from build123d import *

# Parameters (mm, degrees)
EXTRUDE_1_DEPTH          = 2.5
EXTRUDE_1_DEPTH_BACK     = 2.5
SKETCH_1_W               = 10
SKETCH_1_H               = 5
EXTRUDE_3_DEPTH          = 1
EXTRUDE_3_DEPTH_BACK     = 1
SKETCH_2_6_R             = 0.5
CUT_EXTRUDE_1_DEPTH      = 0.5
CUT_EXTRUDE_1_DEPTH_BACK = 0.5
SKETCH_2_R               = 0.5


with BuildPart() as part:
    # Sketch 1 → Extrude 1 (new, two sides: drawn at the far end of the back side and taken through both)
    with BuildSketch(Plane.XY.offset(-EXTRUDE_1_DEPTH_BACK)):
        with Locations((5, 2.5)):
            Rectangle(SKETCH_1_W, SKETCH_1_H)
    extrude(amount=EXTRUDE_1_DEPTH + EXTRUDE_1_DEPTH_BACK)

    # Sketch 2_6 → Extrude 3 (add, two sides: drawn at the far end of the back side and taken through both)
    with BuildSketch(Plane.XY.offset(-EXTRUDE_3_DEPTH_BACK)):
        with BuildLine():
            Line((3.5, 5), (6.5, 5))
            ThreePointArc((6.5, 5), (5.969669914, 5.219669914), (5.75, 5.75))
            ThreePointArc((5.75, 5.75), (5, 6.5), (4.25, 5.75))
            ThreePointArc((4.25, 5.75), (4.030330086, 5.219669914), (3.5, 5))
        make_face()
        with Locations((5, 5.75)):
            Circle(SKETCH_2_6_R, mode=Mode.SUBTRACT)
    extrude(amount=EXTRUDE_3_DEPTH + EXTRUDE_3_DEPTH_BACK)

    # Sketch 2 → Cut-Extrude 1 (cut, two sides: drawn at the far end of the back side and taken through both)
    with BuildSketch(Plane.XY.offset(-CUT_EXTRUDE_1_DEPTH_BACK)):
        with BuildLine():
            Line((3.5, 5), (6.5, 5))
            ThreePointArc((6.5, 5), (5.969669914, 5.219669914), (5.75, 5.75))
            ThreePointArc((5.75, 5.75), (5, 6.5), (4.25, 5.75))
            ThreePointArc((4.25, 5.75), (4.030330086, 5.219669914), (3.5, 5))
        make_face()
        with Locations((5, 5.75)):
            Circle(SKETCH_2_R, mode=Mode.SUBTRACT)
    extrude(amount=CUT_EXTRUDE_1_DEPTH + CUT_EXTRUDE_1_DEPTH_BACK, mode=Mode.SUBTRACT)


solid = part.part
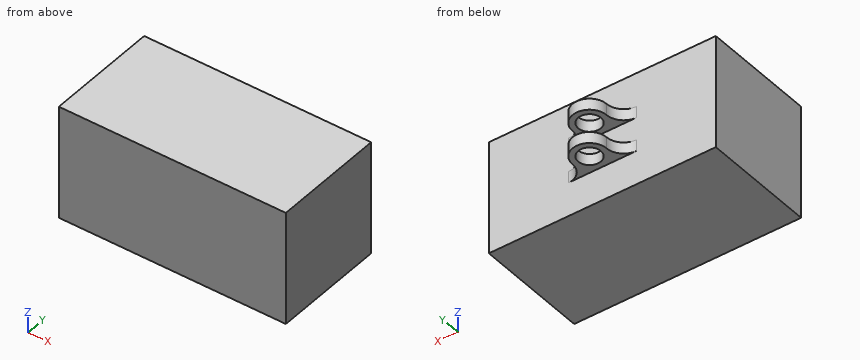
Verification items for the finished model (mm, model axes). Give positions to 0.01 mm unless a question says otherwise; leave off trailing zeros. Write each loop counter-clockwise with the first axis right and the second up, starting at its lowest first coordinate (ties: lowest second). Pieces come first, ordered by that corner, then holes. Notation, with made-up numbers: M -14,-38.75 L 31,-38.75 A28 cw 31,-13.75 Z; hole C 47,80 d4. An arc over 180 degrees is marked long. Write item = value, one per line.
(1) Sectioned sample at D-D (z = 2.25). Record the cut outline in (x, y).
Found:
outline = M 0,0 L 10,0 L 10,5 L 0,5 Z
(2) Sectioned sample at C-C (y = 5.5). Record the cut outline in (x, z).
Found:
outline = M 4.21,-1 L 4.57,-1 L 4.57,-0.5 L 4.21,-0.5 Z; M 4.21,0.5 L 4.57,0.5 L 4.57,1 L 4.21,1 Z; M 5.43,-1 L 5.79,-1 L 5.79,-0.5 L 5.43,-0.5 Z; M 5.43,0.5 L 5.79,0.5 L 5.79,1 L 5.43,1 Z
(3) Sectioned sample at B-B (z = 0.7). Record the cut outline in (x, y), then the cut area to 3 significant figures.
Found:
outline = M 0,0 L 10,0 L 10,5 L 6.5,5 A0.75 cw 5.75,5.75 A0.75 ccw 4.25,5.75 A0.75 cw 3.5,5 L 0,5 Z; hole C 5,5.75 d1
area = 51.5 mm2
(4) Go/stop test with flat-tipped pins: pin 1 Ø3 at (x, z) = (2.5, 2) entering from +Y; pin 2 Ø0.8 at (x, y) = (5, 6) entering from +Z. Record where each tip stops, or that it passes through.
Found:
pin_1 = 5.01
pin_2 = 1
(5) Material ranges on line 1 (Z direction, x = 5.75, y = 5.5); line 2 (Y direction, x = 1, z = 2.25); line 3 (X direction, y = 6, z = 0.55), recorded low to high.
Found:
line_1 = -1 to -0.5, 0.5 to 1
line_2 = 0 to 5
line_3 = 4.29 to 4.57, 5.43 to 5.71
(6) Sectioned sample at A-A (x = 5). Record the cut outline in (y, z), then the cut area to 3 significant figures.
Found:
outline = M 0,-2.5 L 5,-2.5 L 5,-1 L 5.25,-1 L 5.25,-0.5 L 5,-0.5 L 5,0.5 L 5.25,0.5 L 5.25,1 L 5,1 L 5,2.5 L 0,2.5 Z; M 6.25,-1 L 6.5,-1 L 6.5,-0.5 L 6.25,-0.5 Z; M 6.25,0.5 L 6.5,0.5 L 6.5,1 L 6.25,1 Z
area = 25.5 mm2
